The model under review builds one solid part; all positions refer to its coordinate system, in mm. A direction names the side the tool comes from. Coordinates: 2 decimals unless noted, no trailing zeros. Write each loop counter-clockwise with the first axis right and the second up, starting at its lowest first coordinate (ties: lowest second). Pieces come first, ordered by that corner, then holes. Notation, with made-up numbers: (86, 57) -> (107, 57) arc R35 cw to (107, 95) -> close; hole circle Ø8 at (43, -15). An arc over 180 degrees is marked (long way). Write each question's results on one line, items separated by ' | '.
```python
from build123d import *

# Parameters (mm, degrees)
SKETCH1_R           = 9.35
SKETCH1_R_2         = 6.35
SKETCH1_R_3         = 5
BOSS_EXTRUDE1_DEPTH = 5
SKETCH1_3_R         = 9.35
SKETCH1_3_R_2       = 6.35
BOSS_EXTRUDE2_DEPTH = 10
SKETCH2_R           = 1.4
CUT_EXTRUDE1_DEPTH  = 10.35


with BuildPart() as part:
    # Sketch1 → Boss-Extrude1 (new body)
    with BuildSketch(Plane(origin=(0, 0, 0), x_dir=(1, 0, 0), z_dir=(0, 1, 0))):
        Circle(SKETCH1_R)
        Circle(SKETCH1_R_2, mode=Mode.SUBTRACT)
        with BuildLine():
            Line((33.520573743, 17.370769583), (-2.1120271, 9.10833912))
            ThreePointArc((-2.1120271, 9.10833912), (5.817002949, 7.320176001), (9.35, 0))
            ThreePointArc((9.35, 0), (5.817002949, -7.320176001), (-2.1120271, -9.10833912))
            Line((-2.1120271, -9.10833912), (33.520573743, -17.370769583))
            ThreePointArc((33.520573743, -17.370769583), (31.539303236, -8.585467379), (39.65, -12.5))
            Line((39.65, -12.5), (39.65, 12.5))
            ThreePointArc((39.65, 12.5), (31.539303236, 8.585467379), (33.520573743, 17.370769583))
        make_face()
        with Locations((34.65, 12.5)):
            Circle(SKETCH1_R_3)
        with Locations((34.65, -12.5)):
            Circle(SKETCH1_R_3)
    extrude(amount=BOSS_EXTRUDE1_DEPTH)

    # Sketch1_3 → Boss-Extrude2 (add)
    with BuildSketch(Plane(origin=(0, 0, 0), x_dir=(1, 0, 0), z_dir=(0, 1, 0))):
        Circle(SKETCH1_3_R)
        Circle(SKETCH1_3_R_2, mode=Mode.SUBTRACT)
    extrude(amount=BOSS_EXTRUDE2_DEPTH)

    # Sketch2 → Cut-Extrude1 (cut, through all)
    with BuildSketch(Plane(origin=(0, 0, 0), x_dir=(0, 0, -1), z_dir=(1, 0, 0))):
        with Locations((0, 5)):
            Circle(SKETCH2_R)
    extrude(amount=-CUT_EXTRUDE1_DEPTH, mode=Mode.SUBTRACT)


solid = part.part
```
Q1. Add section D-D (z = -8). Write out the cut boundary in (x, y), plus the area to 3 significant figures.
Solution:
outline: (-4.84, 0) -> (39.65, 0) -> (39.65, 5) -> (4.84, 5) -> (4.84, 10) -> (-4.84, 10) -> close | area: 271 mm²
Q2. Add section B-B (x = 0). Write out the cut boundary in (y, z), plus the area to 3 significant figures.
Solution:
outline: (0, -9.6) -> (5, -9.6) -> (5, -9.35) -> (10, -9.35) -> (10, -6.35) -> (0, -6.35) -> close; (0, 6.35) -> (10, 6.35) -> (10, 9.35) -> (5, 9.35) -> (5, 9.6) -> (0, 9.6) -> close | area: 62.5 mm²
Q3. Clearance check with flat-ended pins moving along their axes: P1, Ø7.5, axis at x = 0, z = 0, coming from the -Y side; P2, Ø8, axis at x = 23, z = 0.5, coming from the +Y side; P3, Ø2, axis at x = 4, y = 7, coming from the +Z side. State where each tip first meets the part, or that it passes through.
Solution:
P1: through | P2: y = 5 | P3: z = 8.86
Q4. Add section A-A (z = 0). Write out the cut boundary in (x, y), plus the area to 3 significant figures.
Solution:
outline: (-9.35, 0) -> (-6.35, 0) -> (-6.35, 3.6) -> (-9.35, 3.6) -> close; (-9.35, 6.4) -> (-6.35, 6.4) -> (-6.35, 10) -> (-9.35, 10) -> close; (6.35, 0) -> (39.65, 0) -> (39.65, 5) -> (9.35, 5) -> (9.35, 10) -> (6.35, 10) -> close | area: 203 mm²
Q5. For line 1 (Y direction, x = -8.1, z = 0); line 2 (Y direction, x = 27, z = 12); line 3 (X direction, y = 3.25, z = -7), list the stretches that pass through material, from the lowest coordinate up. Write a range as from..to.
Solution:
line 1: 0..3.6, 6.4..10 | line 2: 0..5 | line 3: -6.2..39.65
Q6. Add section C-C (y = 2.75). Write out the cut boundary in (x, z).
Solution:
outline: (-2.11, -9.11) -> (33.52, -17.37) arc R5 ccw to (39.65, -12.5) -> (39.65, 12.5) arc R5 ccw to (33.52, 17.37) -> (-2.11, 9.11) arc R9.35 ccw to start; hole circle Ø12.7 at (0, 0)
Q7. Draft analysis for pull direction X (two halves, no side actions). For faces 3 (the cylindrical face through (6.057, 4.93, -1.907)), 4 (the flat face through (39.65, 2, 0)), 5 (the cylindrical face through (-7.75, 3.76, -0.65)), 6 (the flat face through (15.45, 2.46, 13.18)), state which applies: pulls with the +X half, pulls with the -X half, needs draft (parallel to the pull), parting line crosses it, or undercut.
Solution:
face 3: undercut | face 4: pulls with the +X half | face 5: needs draft | face 6: pulls with the -X half
Q8. Machinability: for faces 1 (the flat face through (15.954, 2.465, -13.297)), 2 (the cylindrical face through (-9.34, 7.15, -0.41)), which of the approach directions +Z, -Z, +X, -X, +Y, -Y give a long, thin tool a straight path to every point of the face, cutting with its end or side? Answer none if there is none.
Solution:
face 1: -Z, -X, +Y, -Y | face 2: +Y
